Design review of the part built by this model. Coordinates are the model's own, in mm. A direction names the side the tool comes from. Coordinates: 2 decimals unless noted, no trailing zeros. Write each loop counter-clockwise with the first axis right and the second up, starting at its lowest first coordinate (ties: lowest second). Pieces come first, ordered by that corner, then holes.
Autodesk Inventor part; units mm, degrees
ref_plane "YZ Plane" through (0, 0, 0) normal (1, 0, 0) x (0, 1, 0)
ref_plane "XZ Plane" through (0, 0, 0) normal (0, 1, 0) x (-1, 0, 0)
ref_plane "XY Plane" through (0, 0, 0) normal (0, 0, 1) x (1, 0, 0)
ref_plane "Arbeitsebene1" through (0, 0, 0) normal (0, 0, 1) x (1, 0, 0)
sketch "Skizze1" plane through (0, 0, 0) normal (0, 0, 1) x (1, 0, 0)
  circle A0 centre (-14.875, 15.5) radius 2.45
  circle A1 centre (-28.2984, -7.75) radius 2.45
  circle A2 centre (-1.4516, -7.75) radius 2.45
  line L0 (-72.925, 40.25) -> (85.125, 40.25)
  line L1 (85.125, -40.25) -> (-72.925, -40.25)
  line L2 (10.125, -40.25) -> (-39.875, -40.25)
  line L3 (-39.875, -40.25) -> (-39.875, 40.25)
  line L4 (-39.875, 40.25) -> (10.125, 40.25)
  line L5 (10.125, 40.25) -> (10.125, -40.25)
  circle A3 centre (-28.2984, -7.75) radius 2.45
  circle A4 centre (-1.4516, -7.75) radius 2.45
  circle A5 centre (-14.875, 15.5) radius 2.45
  point P0 (0, 0)
  dimension "d4" = 25
  dimension "d5" = 50
extrude "Extrusion1" add sketch "Skizze1" along normal blind 10
ref_plane "Arbeitsebene2" through (-39.875, 40.25, 0) normal (0, 1, 0) x (1, 0, 0)
sketch "Skizze4" plane through (-39.875, 40.25, 0) normal (0, 1, 0) x (1, 0, 0)
  line L0 (50, 0) -> (50, -10)
  line L1 (50, -10) -> (50, 18)
  line L2 (50, 18) -> (-48.05, 18)
  line L3 (-48.05, 18) -> (-48.05, 2)
  line L4 (-48.05, 2) -> (8, 2)
  line L5 (8, 2) -> (8, -10)
  line L6 (50, -10) -> (0, -10)
  line L7 (50, -10) -> (8, -10)
  line L8 (-48.05, -54) -> (-48.05, 13)
  point P0 (39.875, 0)
  dimension "d15" = 28
  dimension "d17" = 90
  dimension "d22" = 0
  dimension "d23" = 98.05
extrude "Extrusion3" add sketch "Skizze4" along normal blind 15
properties part number "Querplattenaufsatz"
(1) Consider section D-D (x = -16). Give the boundary of the cut face in (y, z).
(2) Consider section B-B (z = 6). Give the boundary of the cut face in (x, y) (3 decimals), plus the area to 3 significant figures.
(3) For faces 5 (the flat face through (-31.875, 48, 4)), 6 (the flat face through (-15, 1, 0)), 7 (the flat face through (-60, 48, -2)), list the 3-axis set-ups (+Z, -Z, +X, -X, +Y, -Y) from which the entire face can be reached by the end or side of a thin tool; tool diameter is ignored.
(4) Consider section C-C (y = -7.75). Give the boundary of the cut face in (x, z) (3 decimals).
(5) Consider section A-A (y = 15.5). Give the boundary of the cut face in (x, z) (3 decimals).
(6) Wall thickness on line 1 (Y direction, x = -62.5, z = -7); line 2 (X direction, y = 8, z = 4.75) (3 decimals); line 3 (Z direction, x = -3, y = -26): over which ranges is each line inside the solid? List them lowest first.
(7) Mouldability with a two-part tool opening along Y and no side actions: class faces 1 (the flat face through (-36, 40.25, 5)), 2 (the cylindrical face through (-25.962, -8.486, 4.93)), 3 (the cylindrical face through (-1.983, -5.358, 4.93)), 4 (the flat face through (-39.875, -1, 5)) as +Y half, -Y half, draft (parallel to the pull), parting line (faces both ways), or undercut.
(8) Insertion check: pin 1 Ø5.5 at (x, y) = (-14.875, 15.5) entering from -Z; pin 2 Ø3.5 at (y, z) = (46, 3) entering from -X (3 decimals); pin 3 Ø4 at (x, y) = (-28.3, -7.75) entering from -Z; pin 4 Ø12 at (x, y) = (-51, 44.5) entering from +Z. Each pin has a flat end and moves straight along its axis. Give the tip position at first contact, or say it passes through.
Results:
1. outline: (-40.25, 0) - (13.32, 0) - (13.32, 10) - (-40.25, 10) - close; (17.68, 0) - (40.25, 0) - (40.25, -18) - (55.25, -18) - (55.25, 10) - (17.68, 10) - close
2. outline: (-39.875, -40.25) - (10.125, -40.25) - (10.125, 55.25) - (-31.875, 55.25) - (-31.875, 40.25) - (-39.875, 40.25) - close; hole circle Ø4.9 at (-28.298, -7.75); hole circle Ø4.9 at (-14.875, 15.5); hole circle Ø4.9 at (-1.452, -7.75)
2. area: 4,600 mm2
3. face 5: +Z, -X, +Y
3. face 6: -Z, +X, -X, -Y
3. face 7: +Z, -X, +Y, -Y
4. outline: (-39.875, 0) - (-30.748, 0) - (-30.748, 10) - (-39.875, 10) - close; (-25.848, 0) - (-3.902, 0) - (-3.902, 10) - (-25.848, 10) - close; (0.998, 0) - (10.125, 0) - (10.125, 10) - (0.998, 10) - close
5. outline: (-39.875, 0) - (-17.325, 0) - (-17.325, 10) - (-39.875, 10) - close; (-12.425, 0) - (10.125, 0) - (10.125, 10) - (-12.425, 10) - close
6. line 1: y = 40.25 to 55.25
6. line 2: x = -39.875 to 10.125
6. line 3: z = 0 to 10
7. face 1: +Y half
7. face 2: undercut
7. face 3: undercut
7. face 4: draft
8. pin 1: stops at z = 0
8. pin 2: stops at x = -31.875
8. pin 3: passes through
8. pin 4: stops at z = -2
